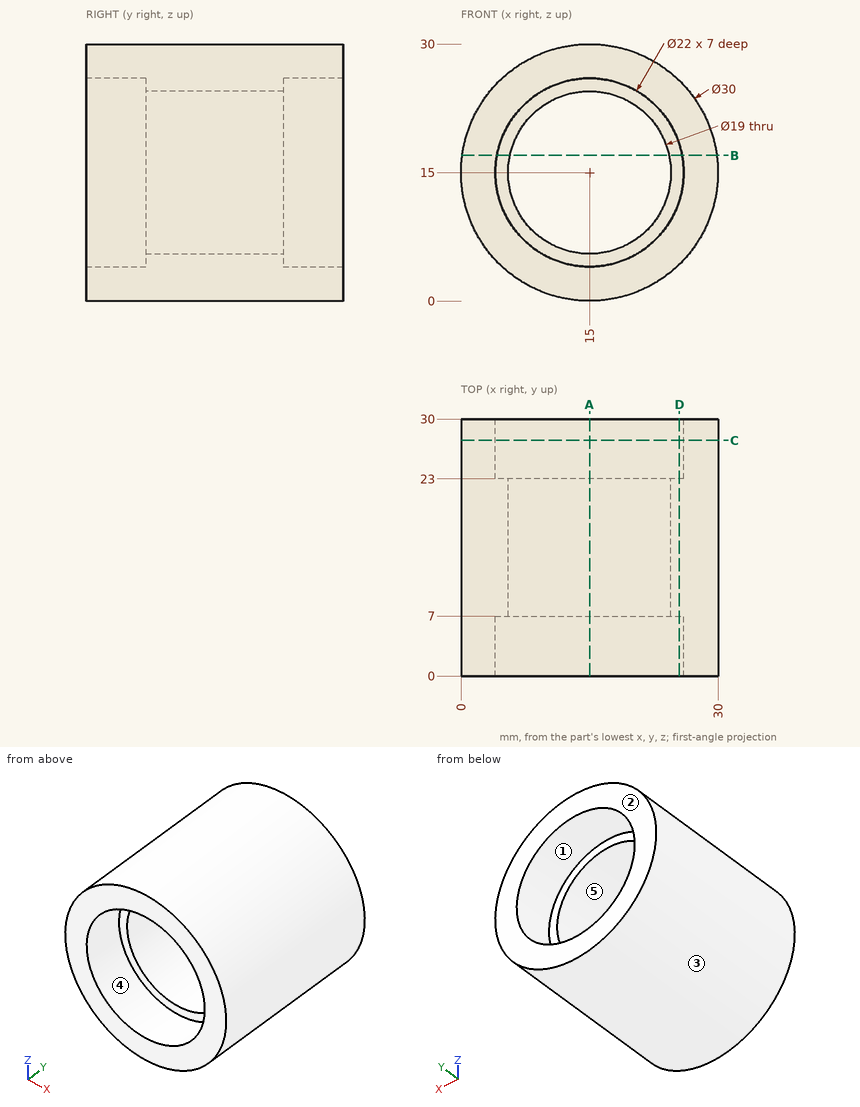
The figure shows three views and two pictorial views of one solid part (mm, origin at its lowest corner). Answer the questions. A direction names the side the tool comes from. Give positions to 0.01 mm unless a question says otherwise; leave off trailing zeros. Order: outer loops, then holes, each group sorted by start corner. A loop starts at its lowest first (then second) coordinate and runs counter-clockwise, first axis right, second up. Notation, with made-up numbers: (-24.75, -24.5) -> (1.25, -24.5) arc R18 cw to (1.25, 7.5) -> close; hole circle Ø9 at (31, -4). An arc over 180 degrees is marked (long way). Answer as a JSON object with one key per item and string values. Group by question number.
Item 1: The part is cut by section C-C on y = 27.5. Write down the section's boundary in (x, z).
Item 2: The part is cut by section A-A on x = 15. Write down the section's boundary in (y, z).
Item 3: Consider L1, parallel to X at y = 5.25, z = 15; L2, parallel to X at y = 13.5, z = 15; L3, parallel to Z at x = 21.75, y = 26.5. Determine where each line is inside the solid, lowest interval first. Write a range as from..to.
Item 4: Flat-ended cylindrical pins translate along their axes: pin 1 (6 mm diameter, centred on x = 6.5, y = 6, fed in from +Z); pin 2 (11 mm diameter, centred on x = 15.5, z = 12.5, fed in from -Y); pin 3 (6 mm diameter, centred on y = 18, z = 3.5, fed in from +X); pin 4 (2 mm diameter, centred on x = 16.5, y = 15, fed in from -Z). Find the tip coordinate at first contact, or state that the pin passes through.
Item 5: The part is cut by section D-D on x = 25.5. Write down the section's boundary in (y, z), and give its area (3 significant figures).
Item 6: The part is cut by section B-B on z = 17. Write down the section's boundary in (x, y).
Item 7: A tool of negligible diameter and unlimited length cuts with its end or side. For the marked faces 4 and 5, from which of +Z, -Z, +X, -X, +Y, -Y can it reach the whole face along a straight path? Write none if from no direction.
Item 8: Determine the mould class of the marked faces 1, 2 and 3 for opening direction X: pulls with the +X half, pulls with the -X half, needs draft (parallel to the pull), parting line crosses it, or undercut.
Result set:
{
 "1": {"outline": "circle Ø30 at (15, 15); hole circle Ø22 at (15, 15)"},
 "2": {"outline": "(0, 0) -> (30, 0) -> (30, 4) -> (23, 4) -> (23, 5.5) -> (7, 5.5) -> (7, 4) -> (0, 4) -> close; (0, 26) -> (7, 26) -> (7, 24.5) -> (23, 24.5) -> (23, 26) -> (30, 26) -> (30, 30) -> (0, 30) -> close"},
 "3": {"L1": "0..4, 26..30", "L2": "0..5.5, 24.5..30", "L3": "1.6..6.31, 23.69..28.4"},
 "4": {"pin 1": "z = 28.96", "pin 2": "through", "pin 3": "x = 27.36", "pin 4": "z = 0.01"},
 "5": {"outline": "(0, 4.29) -> (30, 4.29) -> (30, 11.72) -> (23, 11.72) -> (23, 18.28) -> (30, 18.28) -> (30, 25.71) -> (0, 25.71) -> (0, 18.28) -> (7, 18.28) -> (7, 11.72) -> (0, 11.72) -> close", "area": "551 mm²"},
 "6": {"outline": "(0.13, 0) -> (4.18, 0) -> (4.18, 7) -> (5.71, 7) -> (5.71, 23) -> (4.18, 23) -> (4.18, 30) -> (0.13, 30) -> close; (24.29, 7) -> (25.82, 7) -> (25.82, 0) -> (29.87, 0) -> (29.87, 30) -> (25.82, 30) -> (25.82, 23) -> (24.29, 23) -> close"},
 "7": {"face 4": "-Y", "face 5": "+Y, -Y"},
 "8": {"face 1": "undercut", "face 2": "needs draft", "face 3": "parting line crosses it"}
}
